```python
from build123d import *

# Parameters (mm, degrees)
F0_R     = 12.5
F1_DEPTH = 10


with BuildPart() as f1:
    # F0 (on Top) → F1 (new body)
    with BuildSketch(Plane.XY):
        with BuildLine():
            ThreePointArc((0, 17.5), (5.1256313292, 5.1256313292), (17.5, 0))
            Line((17.5, 0), (78, 0))
            ThreePointArc((78, 0), (81.5355339059, 1.4644660941), (83, 5))
            Line((83, 5), (83, 36.5))
            ThreePointArc((83, 36.5), (81.5355339059, 40.0355339059), (78, 41.5))
            Line((78, 41.5), (17.5, 41.5))
            ThreePointArc((17.5, 41.5), (5.1256313292, 36.3743686708), (0, 24))
            Line((0, 24), (0, 17.5))
        make_face()
        with Locations((17.5, 21)):
            Circle(F0_R, mode=Mode.SUBTRACT)
    extrude(amount=F1_DEPTH)

    # F3 (on offset) → F4 (revolve, cut)
    with BuildSketch(Plane.XY.offset(10.5)):
        Polygon((44.5, 27), (44.5, 2), (49, 2), (49, 27), (54, 27), (54, 34.5), (51.5, 34.5), (51.5, 39.5), (44.5, 39.5), (44.5, 34.5), align=None)
    revolve(axis=Axis((44.5, 14.5, 10.5), (0, 1, 0)), mode=Mode.SUBTRACT)

    # F3 (on offset) → F5 (revolve, cut)
    with BuildSketch(Plane.XY.offset(10.5)):
        Polygon((68.5, 27), (68.5, 2), (73, 2), (73, 27), (78, 27), (78, 34.5), (75.5, 34.5), (75.5, 39.5), (68.5, 39.5), (68.5, 34.5), align=None)
    revolve(axis=Axis((68.5, 14.5, 10.5), (0, 1, 0)), mode=Mode.SUBTRACT)


solid = f1.part
```
Geometry check sheet. Reference: the model listing, model coordinates, mm. A direction names the side the tool comes from. Round coordinates to 2 decimals unless told otherwise and drop trailing zeros. Order: outer loops, then holes, each group sorted by start corner. A loop starts at its lowest first (then second) coordinate and runs counter-clockwise, first axis right, second up. Notation, with made-up numbers: (4.5, 73.25) -> (16.5, 73.25) arc R17 ccw to (16.5, 106.25) -> close; hole circle Ø1 at (78, 82.5). An arc over 180 degrees is marked (long way). Return JSON: item names as keys, results as strings. Group by question number.
Q1. Tool access check on faces 1 (the flat face through (41, 21, 0)), 2 (the flat face through (68, 39.5, 7)). Record the directions out of +Z, -Z, +X, -X, +Y, -Y that give a thin tool (end or side, any length) a straight path to the whole face; none if there is none.
Q2. Section check C-C, the plane z = 2.25. Record the boundary of the cut face in (x, y), plus the area to 3 significant figures.
Q3. Release check for a two-part mould opening along Y. For faces 3 (the cylindrical face through (44.6, 14.7, 6)), 4 (the cylindrical face through (5.26, 36.51, 4.93)), 5 (the flat face through (0, 21, 5)), 6 (the cylindrical face through (81, 1, 5)) record: released by +Y, released by -Y, zero draft, split by the parting line, or undercut.
Q4. Section check D-D, the plane x = 68.5. Record the boundary of the cut face in (y, z).
Q5. Material ranges on probe 1 along Y at (x, z) = (52, 6.5); probe 2 along Y at (x, z) = (17.5, 6); probe 3 along X at (y, z) = (28, 3.75), recorded low to high. Write a range as from..to.
Q6. Section check A-A, the plane y = 21. Record the boundary of the cut face in (x, z).
Q7. Section check B-B, the plane x = 10. Record the boundary of the cut face in (y, z).
Q8. Gauge pin test, flat ends, axial feed: pin 1 (6 mm diameter, centred on y = 31, z = 9, fed in from -X); pin 2 (22.5 mm diameter, centred on x = 17.5, y = 21, fed in from +Z). Record the tip position at first contact, or that the pin passes through.
Numbers:
{
 "1": {"face 1": "-Z, +X, -X, +Y, -Y", "face 2": "+Z"},
 "2": {"outline": "(0, 17.5) arc R17.5 ccw to (17.5, 0) -> (78, 0) arc R5 ccw to (83, 5) -> (83, 36.5) arc R5 ccw to (78, 41.5) -> (17.5, 41.5) arc R17.5 ccw to (0, 24) -> close; hole circle Ø25 at (17.5, 21); hole (39.79, 27) -> (49.21, 27) -> (49.21, 34.5) -> (39.79, 34.5) -> close; hole (63.79, 27) -> (73.21, 27) -> (73.21, 34.5) -> (63.79, 34.5) -> close", "area": "2,670 mm^2"},
 "3": {"face 3": "undercut", "face 4": "released by +Y", "face 5": "zero draft", "face 6": "released by -Y"},
 "4": {"outline": "(0, 0) -> (41.5, 0) -> (41.5, 10) -> (39.5, 10) -> (39.5, 3.5) -> (34.5, 3.5) -> (34.5, 1) -> (27, 1) -> (27, 6) -> (2, 6) -> (2, 10) -> (0, 10) -> close"},
 "5": {"probe 1": "0..27, 34.5..41.5", "probe 2": "0..8.5, 33.5..41.5", "probe 3": "0.46..7.14, 27.86..37.82, 51.18..61.82, 75.18..83"},
 "6": {"outline": "(0, 0) -> (5, 0) -> (5, 10) -> (0, 10) -> close; (30, 0) -> (83, 0) -> (83, 10) -> (72.97, 10) arc R4.5 cw to (64.03, 10) -> (48.97, 10) arc R4.5 cw to (40.03, 10) -> (30, 10) -> close"},
 "7": {"outline": "(1.69, 0) -> (11, 0) -> (11, 10) -> (1.69, 10) -> close; (31, 0) -> (39.81, 0) -> (39.81, 10) -> (31, 10) -> close"},
 "8": {"pin 1": "x = 0.46", "pin 2": "through"}
}
